Work out the finished part from the listing and answer in its coordinate system (mm). A direction names the side the tool comes from. Round coordinates to 2 decimals unless told otherwise and drop trailing zeros. Loops run counter-clockwise (first coordinate to the right, second up) from the corner with the lowest first, then second, coordinate; pieces in that order, holes last. Notation, with made-up numbers: (35, 70.25) - (49, 70.25) arc R31 ccw to (49, 103.25) - close; hole circle Ø9 at (84, -4.5). An arc over 180 degrees is marked (long way). Use CSV: the item, a comma, the result in double quotes. Start each with the question number.
from build123d import *

# Parameters (mm, degrees)
SKETCH1_W               = 200
SKETCH1_H               = 150
BOSS_EXTRUDE1_DEPTH     = 10
CUT_EXTRUDE1_DEPTH      = 214.834047803
CUT_EXTRUDE1_DEPTH_BACK = 214.834047803
SKETCH2_R               = 2.5
SKETCH3_W               = 200
SKETCH3_H               = 3
BOSS_EXTRUDE2_DEPTH     = 60


with BuildPart() as part:
    # Sketch1 → Boss-Extrude1 (new body)
    with BuildSketch(Plane.XY):
        Rectangle(SKETCH1_W, SKETCH1_H)
    extrude(amount=BOSS_EXTRUDE1_DEPTH)

    # Sketch2 → Cut-Extrude1 (cut, two sides: drawn at the far end of the back side and taken through both)
    with BuildSketch(Plane.ZY.offset(100).offset(-CUT_EXTRUDE1_DEPTH_BACK)):
        with Locations((4.560099843, -45.856552044)):
            Circle(SKETCH2_R)
    extrude(amount=CUT_EXTRUDE1_DEPTH + CUT_EXTRUDE1_DEPTH_BACK, mode=Mode.SUBTRACT)

    # Sketch3 → Boss-Extrude2 (add)
    with BuildSketch(Plane.XY.offset(10)):
        with Locations((0, 73.5)):
            Rectangle(SKETCH3_W, SKETCH3_H)
    extrude(amount=BOSS_EXTRUDE2_DEPTH)


solid = part.part
Item 1: Each of these flat-tipped pins is pushed along its axis until it touches: pin 1 Ø1 at (x, z) = (-18, 25.5) entering from -Y; pin 2 Ø8 at (x, y) = (-65.5, -29) entering from +Z; pin 3 Ø4 at (y, z) = (-45.86, 4.56) entering from -X. Where does it stop, or does it pass through?
Item 2: A cutting plane is placed at B-B (z = 29.5). Determine the outline of the cut face in (x, y).
Item 3: Find the intervals of material crossed by probe 1 along Z at (x, y) = (15.5, 34); probe 2 along Y at (x, z) = (31.5, 32), in increasing order. Write a range as [from, to].
Item 4: A cutting plane is placed at A-A (x = 62). Determine the outline of the cut face in (y, z).
Item 5: A cutting plane is placed at C-C (y = 31). Determine the outline of the cut face in (x, z).
Item 6: Which of the six approach directions +Z, -Z, +X, -X, +Y, -Y give full straight-line access (tool end or side, diameter ignored) to faces 4 (the flat face through (-1, 72, 40)), 5 (the flat face through (-100, 0, 6))?
Item 7: The mould has two halves that part along Y. Classify faces 1 (the flat face through (-1, -75, 5)), 2 (the cylindrical face through (1.4, -43.749, 5.904)), 3 (the flat face through (-1, 0, 10)): pulls with the +Y half, pulls with the -Y half, needs draft (parallel to the pull), parting line crosses it, or undercut.
Result sheet:
1,pin 1,"y = 72"
1,pin 2,"z = 10"
1,pin 3,"through"
2,outline,"(-100, 72) - (100, 72) - (100, 75) - (-100, 75) - close"
3,probe 1,"[0, 10]"
3,probe 2,"[72, 75]"
4,outline,"(-75, 0) - (75, 0) - (75, 70) - (72, 70) - (72, 10) - (-75, 10) - close; hole circle Ø5 at (-45.86, 4.56)"
5,outline,"(-100, 0) - (100, 0) - (100, 10) - (-100, 10) - close"
6,face 4,"+Z, +X, -X, -Y"
6,face 5,"+Z, -Z, -X, +Y, -Y"
7,face 1,"pulls with the -Y half"
7,face 2,"undercut"
7,face 3,"needs draft"
